Design review of the part built by this model. Coordinates are the model's own, in mm. A direction names the side the tool comes from. Give positions to 0.01 mm unless a question says otherwise; leave off trailing zeros. Order: outer loops, then holes, each group sorted by start corner. A loop starts at its lowest first (then second) coordinate and runs counter-clockwise, first axis right, second up. Notation, with made-up numbers: (78.25, 25) -> (123.25, 25) arc R16 cw to (123.25, 55) -> close; hole circle Ø11 at (6, 63.25). An arc over 180 degrees is marked (long way). Answer in a Markdown table with one row per item. Add a question column.
```python
from build123d import *

# Parameters (mm, degrees)
CROQUIS1_R                                           = 1.7
SALIENTE_EXTRUIR1_DEPTH                              = 5
CROQUIS11_R                                          = 1.6
CORTAR_EXTRUIR1_DEPTH                                = 6
CORTAR_EXTRUIR2_REACH                                = 141.352
CROQUIS13_R                                          = 1.8
SALIENTE_EXTRUIR2_DEPTH                              = 2
SALIENTE_EXTRUIR3_START                              = -0.5
CROQUIS13_3_R                                        = 4
CROQUIS13_3_R_2                                      = 1.8
SALIENTE_EXTRUIR3_DEPTH                              = 0.5
CORTAR_EXTRUIR3_START                                = -1.5
CROQUIS14_R                                          = 4
CORTAR_EXTRUIR3_DEPTH                                = 1.5
CHAFL_N1_SIZE                                        = 1
REFRENTADO_PARA_TORNILLO_CON_CABEZA_TRON_D           = 3.4
REFRENTADO_PARA_TORNILLO_CON_CABEZA_TRON_CBORE_D     = 5.5
REFRENTADO_PARA_TORNILLO_CON_CABEZA_TRON_CBORE_DEPTH = 1
REDONDEO1_R                                          = 10
REDONDEO2_R                                          = 6


with BuildPart() as part:
    # Croquis1 → Saliente-Extruir1 (new body)
    with BuildSketch(Plane.XY):
        with BuildLine():
            Line((-24.90015137, 109.767857143), (-14.940090822, -1.339285714))
            ThreePointArc((-14.940090822, -1.339285714), (0, -15), (14.940090822, -1.339285714))
            Line((14.940090822, -1.339285714), (24.90015137, 109.767857143))
            ThreePointArc((24.90015137, 109.767857143), (0, 137), (-24.90015137, 109.767857143))
        make_face()
        Circle(CROQUIS1_R, mode=Mode.SUBTRACT)
        with BuildLine():
            ThreePointArc((0, 79.505), (-2.580939751, 80.574060249), (-3.65, 83.155))
            Line((-3.65, 83.155), (-3.65, 101.040870244))
            ThreePointArc((-3.65, 101.040870244), (-4.216609288, 104.359173979), (-5.852227935, 107.30144137))
            ThreePointArc((-5.852227935, 107.30144137), (-6.655195316, 115.468919185), (0.5, 119.488325914))
            ThreePointArc((0.5, 119.488325914), (5.480762949, 117.127013019), (7.505, 112))
            ThreePointArc((7.505, 112), (7.079759729, 109.509613047), (5.852227935, 107.30144137))
            ThreePointArc((5.852227935, 107.30144137), (4.216609288, 104.359173979), (3.65, 101.040870244))
            Line((3.65, 101.040870244), (3.65, 83.155))
            ThreePointArc((3.65, 83.155), (2.580939751, 80.574060249), (0, 79.505))
        make_face(mode=Mode.SUBTRACT)
    extrude(amount=SALIENTE_EXTRUIR1_DEPTH)

    # Croquis11 → Cortar-Extruir1 (cut)
    with BuildSketch(Plane(origin=(0, 0, 0), x_dir=(-1, 0, 0), z_dir=(0, 0, -1))):
        with Locations((-15.5, 64.768083746)):
            Circle(CROQUIS11_R)
        with Locations(Location((15.5, 64.768083746, 0), (0, 0, 180))):
            Circle(CROQUIS11_R)
    extrude(amount=-CORTAR_EXTRUIR1_DEPTH, mode=Mode.SUBTRACT)

    # Croquis12 → Cortar-Extruir2 (cut, up to next)
    with BuildSketch(Plane.XY.offset(5), mode=Mode.PRIVATE) as cortar_extruir2_sk1:
        Polygon((-12, 58), (12, 58), (7.517812675, 8), (-7.517812675, 8), align=None)
    cortar_extruir2_tool1 = extrude(cortar_extruir2_sk1.sketch, amount=-CORTAR_EXTRUIR2_REACH, mode=Mode.PRIVATE) & part.part
    add(cortar_extruir2_tool1.solids().sort_by_distance((0, 34.913717, 5))[0], mode=Mode.SUBTRACT)

    # Croquis13 → Saliente-Extruir2 (add)
    with BuildSketch(Plane.XY.offset(5)):
        with BuildLine():
            Line((6.784704059, 84.864496193), (9.143753072, 111.180319718))
            ThreePointArc((9.143753072, 111.180319718), (0, 121.180419163), (-9.143753072, 111.180319718))
            Line((-9.143753072, 111.180319718), (-6.784704059, 84.864496193))
            ThreePointArc((-6.784704059, 84.864496193), (0, 78.660792028), (6.784704059, 84.864496193))
        make_face()
        with Locations((0, 112)):
            Circle(CROQUIS13_R, mode=Mode.SUBTRACT)
    extrude(amount=SALIENTE_EXTRUIR2_DEPTH)

    # Croquis13<3> → Saliente-Extruir3 (add)
    with BuildSketch(Plane.XY.offset(5).offset(SALIENTE_EXTRUIR3_START)):
        with Locations((0, 112)):
            Circle(CROQUIS13_3_R)
        with Locations((0, 112)):
            Circle(CROQUIS13_3_R_2, mode=Mode.SUBTRACT)
    extrude(amount=SALIENTE_EXTRUIR3_DEPTH)

    # Croquis14 → Cortar-Extruir3 (cut)
    with BuildSketch(Plane.XY.offset(7).offset(CORTAR_EXTRUIR3_START)):
        with Locations((0, 112)):
            Circle(CROQUIS14_R)
    extrude(amount=CORTAR_EXTRUIR3_DEPTH, mode=Mode.SUBTRACT)

    # Chaflán1
    chafl_n1_edges = [part.edges().sort_by_distance(p)[0] for p in [
        (3.65, 92.097935122, 0),
        (4.216609288, 104.359173979, 0),
        (-2.490386953, 119.079759729, 0),
        (-4.216609288, 104.359173979, 0),
        (-3.65, 92.097935122, 0),
        (0, 79.505, 0),
    ]]
    chamfer(chafl_n1_edges, length=CHAFL_N1_SIZE)

    # Refrentado para tornillo con cabeza troncocónica de M31 (through all)
    with Locations(Plane(origin=(0, 0, 7), x_dir=(-1, 0, 0), z_dir=(0, 0, 1))):
        with Locations((0, -91.915), (0, -87.915)):
            CounterBoreHole(REFRENTADO_PARA_TORNILLO_CON_CABEZA_TRON_D / 2, REFRENTADO_PARA_TORNILLO_CON_CABEZA_TRON_CBORE_D / 2, REFRENTADO_PARA_TORNILLO_CON_CABEZA_TRON_CBORE_DEPTH)

    # Redondeo1
    redondeo1_edges = [part.edges().sort_by_distance(p)[0] for p in [
        (-1.887458609, 89.915, 6.5),
        (1.887458609, 89.915, 6.5),
    ]]
    fillet(redondeo1_edges, radius=REDONDEO1_R)

    # Redondeo2
    redondeo2_edges = [part.edges().sort_by_distance(p)[0] for p in [
        (7.517812675, 8, 2.5),
        (-7.517812675, 8, 2.5),
        (-12, 58, 2.5),
        (12, 58, 2.5),
    ]]
    fillet(redondeo2_edges, radius=REDONDEO2_R)


solid = part.part
```
1) Add section A-A, the plane y = 0. Write out the cut boundary in (x, z).
2) Clearance check with flat-ended pins moving along their axes: P1, Ø1.2, axis at x = -1, z = 2, coming from the +Y side; P2, Ø2.5, axis at x = 0, y = 114, coming from the +Z side; P3, Ø25, axis at x = 5.5, y = 59, coming from the +Z side; P4, Ø12, axis at x = 5, y = 25, coming from the -Z side. State where each tip first meets the part, or that it passes through.
3) Machinability: for faces 1 (the face through (-4.2, 104.31, 2.97)), 2 (the face through (-9.687, 32.198, 2.535)), 3 (the face through (5, 79, 0)), 4 (the face through (-0.067, 85.166, 6.507)), which of the approach directions +Z, -Z, +X, -X, +Y, -Y give a long, thin tool a straight path to every point of the face, cutting with its end or side? Answer none if there is none.
4) For L1, parallel to Y at x = 0, z = 1.8 (3 decimals); L2, parallel to Y at x = 0, z = 6.8 (3 decimals); L3, parallel to Y at x = -6.5, z = 3.25, list the stretches that pass through material, from the lowest coordinate up.
5) Mouldability with a two-part tool opening along Y and no side actions: class faces 5 (the face through (19.85, 53.44, 2.46)), 6 (the face through (-9.91, 56, 2.46)), 7 (the face through (5, 79, 5)) as +Y half, -Y half, draft (parallel to the pull), parting line (faces both ways), or undercut.
Verdict:
| question | item | result |
|---|---|---|
| 1 | outline | (-15.06, 0) -> (-1.7, 0) -> (-1.7, 5) -> (-15.06, 5) -> close; (1.7, 0) -> (15.06, 0) -> (15.06, 5) -> (1.7, 5) -> close |
| 2 | P1 | stops at y = 137 |
| 2 | P2 | stops at z = 5.5 |
| 2 | P3 | stops at z = 5 |
| 2 | P4 | stops at z = 0 |
| 3 | face 1 | -Z |
| 3 | face 2 | +Z, -Z |
| 3 | face 3 | -Z, +X, -X, +Y, -Y |
| 3 | face 4 | +Z |
| 4 | L1 | y = -15 to -1.7, 1.7 to 8, 58 to 79.505, 119.505 to 137 |
| 4 | L2 | y = 78.661 to 85.165, 94.665 to 108, 116 to 121.18 |
| 4 | L3 | y = -13.52 to 10, 57.91 to 108.25, 115.75 to 136.14 |
| 5 | face 5 | -Y half |
| 5 | face 6 | undercut |
| 5 | face 7 | draft |
